Read the model definition and answer for the solid it produces. Units are mm, in the model's axes. A direction names the side the tool comes from. Round coordinates to 2 decimals unless told otherwise and drop trailing zeros. Loops run counter-clockwise (first coordinate to the right, second up) from the corner with the lowest first, then second, coordinate; pieces in that order, holes last. Notation, with made-up numbers: (78, 37) -> (99, 37) arc R29 ccw to (99, 75) -> close; hole circle Ø1 at (26, -7.5). An arc over 180 degrees is marked (long way). Put each result on its own line as item: value.
from build123d import *

# Parameters (mm, degrees)
SKETCH1_W           = 70
SKETCH1_H           = 35
BOSS_EXTRUDE1_DEPTH = 10
SKETCH2_R           = 1.65
CUT_EXTRUDE1_DEPTH  = 10
CUT_EXTRUDE2_DEPTH  = 10
SKETCH4_R           = 2.25
CUT_EXTRUDE3_DEPTH  = 10


with BuildPart() as part:
    # Sketch1 → Boss-Extrude1 (new body)
    with BuildSketch(Plane(origin=(0, 0, 0), x_dir=(1, 0, 0), z_dir=(0, 1, 0))):
        Rectangle(SKETCH1_W, SKETCH1_H)
    extrude(amount=BOSS_EXTRUDE1_DEPTH)

    # Sketch2 → Cut-Extrude1 (cut)
    with BuildSketch(Plane.XY.offset(17.5)):
        with Locations((-23, 5)):
            Circle(SKETCH2_R)
        with Locations((0, 5)):
            Circle(SKETCH2_R)
        with Locations(Location((23, 5, 0), (0, 0, 180))):
            Circle(SKETCH2_R)
    cut_extrude1 = extrude(amount=-CUT_EXTRUDE1_DEPTH, mode=Mode.SUBTRACT)

    # Sketch3 → Cut-Extrude2 (cut)
    with BuildSketch(Plane(origin=(0, 10, 0), x_dir=(1, 0, 0), z_dir=(0, 1, 0))):
        with BuildLine():
            Line((-12.5, 7.5), (12.5, 7.5))
            ThreePointArc((12.5, 7.5), (20, 0), (12.5, -7.5))
            Line((12.5, -7.5), (-12.5, -7.5))
            ThreePointArc((-12.5, -7.5), (-20, 0), (-12.5, 7.5))
        make_face()
    extrude(amount=-CUT_EXTRUDE2_DEPTH, mode=Mode.SUBTRACT)

    # Sketch4 → Cut-Extrude3 (cut)
    with BuildSketch(Plane(origin=(0, 10, 0), x_dir=(1, 0, 0), z_dir=(0, 1, 0))):
        with Locations(Location((-30, -5, 0), (0, 0, 270))):
            Circle(SKETCH4_R)
        with Locations(Location((-30, 5, 0), (0, 0, 90))):
            Circle(SKETCH4_R)
        with Locations(Location((30, -5, 0), (0, 0, 90))):
            Circle(SKETCH4_R)
        with Locations(Location((30, 5, 0), (0, 0, 270))):
            Circle(SKETCH4_R)
    extrude(amount=-CUT_EXTRUDE3_DEPTH, mode=Mode.SUBTRACT)

    # Mirror1: Cut-Extrude1 across plane
    add(cut_extrude1.mirror(Plane.XY), mode=Mode.SUBTRACT)


solid = part.part
Item 1: The part is cut by section D-D (x = -9). Determine the outline of the cut face in (y, z).
Derived:
outline: (0, -17.5) -> (10, -17.5) -> (10, -7.5) -> (0, -7.5) -> close; (0, 7.5) -> (10, 7.5) -> (10, 17.5) -> (0, 17.5) -> close
Item 2: The part is cut by section A-A (x = 0). Determine the outline of the cut face in (y, z), then the cut area to 3 significant figures.
Derived:
outline: (0, -17.5) -> (3.35, -17.5) -> (3.35, -7.5) -> (0, -7.5) -> close; (0, 7.5) -> (3.35, 7.5) -> (3.35, 17.5) -> (0, 17.5) -> close; (6.65, -17.5) -> (10, -17.5) -> (10, -7.5) -> (6.65, -7.5) -> close; (6.65, 7.5) -> (10, 7.5) -> (10, 17.5) -> (6.65, 17.5) -> close
area: 134 mm^2
Item 3: Find the intervals of material crossed by line 1 along Z through (x, y) = (-2.5, 7); line 2 along X through (y, z) = (7.5, 5); line 3 along Y through (x, z) = (-23, 14), in increasing order.
Derived:
line 1: z = -17.5 to -7.5, 7.5 to 17.5
line 2: x = -35 to -32.25, -27.75 to -18.09, 18.09 to 27.75, 32.25 to 35
line 3: y = 0 to 3.35, 6.65 to 10
Item 4: The part is cut by section B-B (y = 1). Determine the outline of the cut face in (x, z).
Derived:
outline: (-35, -17.5) -> (35, -17.5) -> (35, 17.5) -> (-35, 17.5) -> close; hole circle Ø4.5 at (-30, -5); hole circle Ø4.5 at (-30, 5); hole (-12.5, -7.5) -> (12.5, -7.5) arc R7.5 ccw to (12.5, 7.5) -> (-12.5, 7.5) arc R7.5 ccw to start; hole circle Ø4.5 at (30, -5); hole circle Ø4.5 at (30, 5)
Item 5: Which of the six approach directions +Z, -Z, +X, -X, +Y, -Y give full straight-line access (tool end or side, diameter ignored) to faces 5 (the flat face through (0, 10, -8)), 6 (the flat face through (-23, 5, 7.5)), 7 (the flat face through (0, 3, 17.5)), 8 (the flat face through (-23, 5, -7.5)), 9 (the cylindrical face through (-20, 5, 0))?
Derived:
face 5: +Z, -Z, +X, -X, +Y
face 6: +Z
face 7: +Z, +X, -X, +Y, -Y
face 8: -Z
face 9: +Y, -Y
Item 6: The part is cut by section C-C (z = 12.5). Determine the outline of the cut face in (x, y).
Derived:
outline: (-35, 0) -> (35, 0) -> (35, 10) -> (-35, 10) -> close; hole circle Ø3.3 at (-23, 5); hole circle Ø3.3 at (0, 5); hole circle Ø3.3 at (23, 5)
Item 7: For a pull along X with two mould halves and no side action, classify faces 1 (the flat face through (35, 5, 0)), 2 (the flat face through (0, 7, -7.5)), 3 (the flat face through (-35, 5, 0)), 4 (the flat face through (0, 0, -8)) as pulls with the +X half, pulls with the -X half, needs draft (parallel to the pull), parting line crosses it, or undercut.
Derived:
face 1: pulls with the +X half
face 2: undercut
face 3: pulls with the -X half
face 4: needs draft
Item 8: Flat-ended cylindrical pins translate along their axes: pin 1 Ø1 at (x, y) = (-22.5, 5.5) entering from +Z; pin 2 Ø1.6 at (x, y) = (23.5, 5) entering from -Z; pin 3 Ø3 at (x, y) = (0, 5) entering from +Z. Find the tip coordinate at first contact, or state that the pin passes through.
Derived:
pin 1: stops at z = 7.5
pin 2: stops at z = -7.5
pin 3: passes through
